from build123d import *

# Parameters (mm, degrees)
SKETCH1_W           = 25.4
SKETCH1_H           = 50.8
SKETCH1_W_2         = 19.05
SKETCH1_H_2         = 44.45
BOSS_EXTRUDE1_DEPTH = 279.4
CUT_EXTRUDE1_DEPTH  = 279.4
SKETCH3_R           = 2.5527
CUT_EXTRUDE2_DEPTH  = 25.4


with BuildPart() as part:
    # Sketch1 → Boss-Extrude1 (new body)
    with BuildSketch(Plane(origin=(0, 0, 0), x_dir=(1, 0, 0), z_dir=(0, 1, 0))):
        with Locations((12.7, 25.4)):
            Rectangle(SKETCH1_W, SKETCH1_H)
        with Locations((12.7, 25.4)):
            Rectangle(SKETCH1_W_2, SKETCH1_H_2, mode=Mode.SUBTRACT)
    extrude(amount=BOSS_EXTRUDE1_DEPTH)

    # Sketch2 → Cut-Extrude1 (cut)
    with BuildSketch(Plane(origin=(25.4, 0, 0), x_dir=(0, 0, -1), z_dir=(1, 0, 0))):
        Polygon((0, 279.4), (50.8, 228.6), (50.8, 279.4), align=None)
    extrude(amount=-CUT_EXTRUDE1_DEPTH, mode=Mode.SUBTRACT)

    # Sketch3 → Cut-Extrude2 (cut)
    with BuildSketch(Plane(origin=(25.4, 0, 0), x_dir=(0, 0, -1), z_dir=(1, 0, 0))):
        with Locations((12.7, 215.9)):
            Circle(SKETCH3_R)
        with Locations((38.1, 215.9)):
            Circle(SKETCH3_R)
        with Locations((25.4, 190.5)):
            Circle(SKETCH3_R)
        with Locations((12.7, 63.5)):
            Circle(SKETCH3_R)
        with Locations((38.1, 63.5)):
            Circle(SKETCH3_R)
        with Locations((25.4, 88.9)):
            Circle(SKETCH3_R)
    extrude(amount=-CUT_EXTRUDE2_DEPTH, mode=Mode.SUBTRACT)


solid = part.part
CAD build for the part. Positions are in the model's coordinates, mm. A direction names the side the tool comes from. Give positions to 0.01 mm unless a question says otherwise; leave off trailing zeros. Loops run counter-clockwise (first coordinate to the right, second up) from the corner with the lowest first, then second, coordinate; pieces in that order, holes last. Notation, with made-up numbers: M 0.5,57 L 16.5,57 A20 ccw 16.5,84 Z; hole C 53.5,51 d11. An arc over 180 degrees is marked long. Write each question's results on one line, items separated by ' | '.
Q1. Probe probe 1 along Z at (x, y) = (24.7, 215.9); probe 2 along Z at (x, y) = (5, 121.5) (3 decimals); probe 3 along Z at (x, y) = (24, 191). List the from-to ranges inside material, lowest first.
Geometry check:
probe 1: z = -50.8 to -40.65, -35.55 to -15.25, -10.15 to 0 | probe 2: z = -50.8 to -47.625, -3.175 to 0 | probe 3: z = -50.8 to -27.9, -22.9 to 0
Q2. Which spindle directions (+Z, -Z, +X, -X, +Y, -Y) get a long thin tool onto all of the face, cutting with end or side? Do faces 4 (the face through (22.225, 136, -25)), 5 (the face through (23.835, 61.008, -37.547)). Say none if no direction does.
Geometry check:
face 4: +Y, -Y | face 5: +X, -X
Q3. Band-saw the part on D-D on y = 69. Write the cut outline in (x, z) (3 decimals).
Geometry check:
outline: M 0,-50.8 L 25.4,-50.8 L 25.4,0 L 0,0 Z; hole M 3.175,-47.625 L 22.225,-47.625 L 22.225,-3.175 L 3.175,-3.175 Z
Q4. Band-saw the part on A-A on z = -38.1. Write the cut outline in (x, y) (3 decimals), and give its area (3 significant figures).
Geometry check:
outline: M 0,0 L 3.175,0 L 3.175,60.947 L 0,60.947 Z; M 0,66.053 L 3.175,66.053 L 3.175,213.347 L 0,213.347 Z; M 0,218.453 L 3.175,218.453 L 3.175,241.3 L 0,241.3 Z; M 22.225,0 L 25.4,0 L 25.4,60.947 L 22.225,60.947 Z; M 22.225,66.053 L 25.4,66.053 L 25.4,213.347 L 22.225,213.347 Z; M 22.225,218.453 L 25.4,218.453 L 25.4,241.3 L 22.225,241.3 Z | area: 1,470 mm²
Q5. Mould opens along Z. For faces 1 (the face through (13, 113, -50.8)), 2 (the face through (0, 138, -25)), 3 (the face through (1.61, 86.635, -26.578)) say: pulls with the +Z half, pulls with the -Z half, needs draft (parallel to the pull), parting line crosses it, or undercut.
Geometry check:
face 1: pulls with the -Z half | face 2: needs draft | face 3: undercut
Q6. Band-saw the part on B-B on x = 10.75. Write the cut outline in (y, z) (3 decimals).
Geometry check:
outline: M 0,-50.8 L 228.6,-50.8 L 231.775,-47.625 L 0,-47.625 Z; M 0,-3.175 L 276.225,-3.175 L 279.4,0 L 0,0 Z
Q7. Band-saw the part on C-C on y = 215.9. Write the cut outline in (x, z) (3 decimals).
Geometry check:
outline: M 0,-50.8 L 25.4,-50.8 L 25.4,-40.653 L 22.225,-40.653 L 22.225,-47.625 L 3.175,-47.625 L 3.175,-40.653 L 0,-40.653 Z; M 0,-35.547 L 3.175,-35.547 L 3.175,-15.253 L 0,-15.253 Z; M 0,-10.147 L 3.175,-10.147 L 3.175,-3.175 L 22.225,-3.175 L 22.225,-10.147 L 25.4,-10.147 L 25.4,0 L 0,0 Z; M 22.225,-35.547 L 25.4,-35.547 L 25.4,-15.253 L 22.225,-15.253 Z
